Print and shaded views of the part. All mm, measured from the part's lowest x, y and z. Coordinates: 2 decimals unless noted, no trailing zeros. Order: outer loops, then holes, each group sorted by start corner. A loop starts at its lowest first (then second) coordinate and runs counter-clockwise, first axis right, second up. Notation, with made-up numbers: M 33,-21 L 78,-21 A35 cw 78,18 Z; hole C -39,-3.5 d11. An arc over 180 degrees is marked long. Use a Markdown table: item, result. Add a question column.
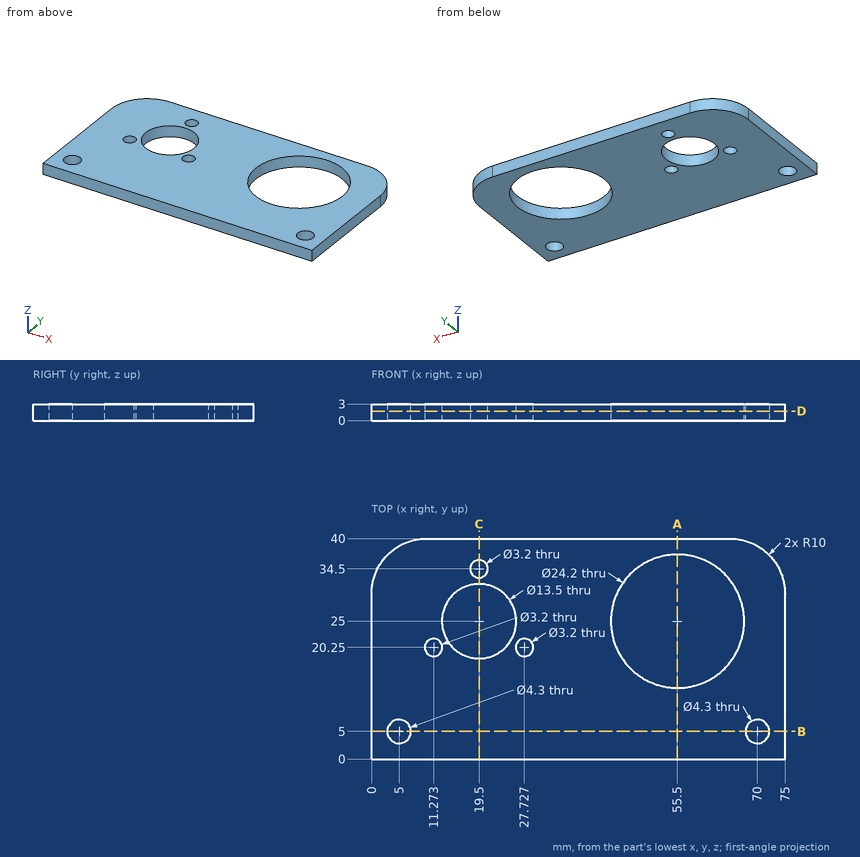
(1) Slice it at A-A on x = 55.5. Give the cut face in (y, z), and give its area (3 significant figures).
(2) Slice it at D-D on z = 1.7. Give the cut face in (x, y), and give its area (3 significant figures).
(3) Slice it at C-C on x = 19.5. Give the cut face in (y, z), and give its area (3 significant figures).
(4) Drill centre lines: line 1 along Y through (x, z) = (19.5, 0.95); line 2 along X through (y, z) = (28, 2.85); line 3 along Y through (x, z) = (55.5, 2.35). Where is each one in solid material? Low to high. Write a range as from..to.
(5) Slice it at B-B on y = 5. Give the cut face in (x, z).
Solutions:
| question | item | result |
|---|---|---|
| 1 | outline | M 0,0 L 12.9,0 L 12.9,3 L 0,3 Z; M 37.1,0 L 40,0 L 40,3 L 37.1,3 Z |
| 1 | area | 47.4 mm² |
| 2 | outline | M 0,0 L 75,0 L 75,30 A10 ccw 65,40 L 10,40 A10 ccw 0,30 Z; hole C 5,5 d4.3; hole C 11.27,20.25 d3.2; hole C 19.5,25 d13.5; hole C 19.5,34.5 d3.2; hole C 27.73,20.25 d3.2; hole C 55.5,25 d24.2; hole C 70,5 d4.3 |
| 2 | area | 2,300 mm² |
| 3 | outline | M 0,0 L 18.25,0 L 18.25,3 L 0,3 Z; M 31.75,0 L 32.9,0 L 32.9,3 L 31.75,3 Z; M 36.1,0 L 40,0 L 40,3 L 36.1,3 Z |
| 3 | area | 69.9 mm² |
| 4 | line 1 | 0..18.25, 31.75..32.9, 36.1..40 |
| 4 | line 2 | 0..13.45, 25.55..43.78, 67.22..75 |
| 4 | line 3 | 0..12.9, 37.1..40 |
| 5 | outline | M 0,0 L 2.85,0 L 2.85,3 L 0,3 Z; M 7.15,0 L 67.85,0 L 67.85,3 L 7.15,3 Z; M 72.15,0 L 75,0 L 75,3 L 72.15,3 Z |
